Geometry check sheet. Reference: the model listing, model coordinates, mm. A direction names the side the tool comes from. Give positions to 0.01 mm unless a question says otherwise; leave off trailing zeros. Loops run counter-clockwise (first coordinate to the right, second up) from the corner with the lowest first, then second, coordinate; pieces in that order, holes last.
1. Cross-section at B-B, the plane y = -11. Record the cut outline in (x, z), plus the area to 3 significant figures.
2. Go/stop test with a flat-tipped pin: pin 1 Ø5 at (y, z) = (2, -0.5) entering from -X. Record where the tip stops, or that it passes through.
3. Cross-section at A-A, the plane x = -0.75. Record the cut outline in (y, z), plus the area to 3 significant figures.
4. Material ranges on L1, parallel to Z at x = 5.75, y = -11; L2, parallel to Z at x = -6.5, y = -8.8; L3, parallel to Y at x = -8.75, z = 3.75, recorded low to high.
5. Tool access check on faces 5 (the cylindrical face through (-5.633, 11.528, -3.905)), 6 (the cylindrical face through (3.79, -9.5, -5.93)), 7 (the flat face through (-5, -9.5, 3)), 8 (the flat face through (4, 13.5, 0)), 9 (the flat face through (0, 0, 0)). Record the directions out of +Z, -Z, +X, -X, +Y, -Y that give a thin tool (end or side, any length) a straight path to the whole face; none if there is none.
6. Cross-section at C-C, the plane z = 6. Record the cut outline in (x, y), plus the area to 3 significant figures.
7. Release check for a two-part mould opening along Y. For faces 1 (the flat face through (-8, 9.5, 3)), 2 (the flat face through (-3, 8.5, 0)), 3 (the flat face through (19, 0, 0)), 4 (the cylindrical face through (3.79, -9.5, 6.07)) record: +Y half, -Y half, draft (parallel to the pull), parting line (faces both ways), or undercut.
8. Cross-section at D-D, the plane x = 8. Record the cut outline in (y, z).
from build123d import *

# Parameters (mm, degrees)
F1_DEPTH = 8.5
F2_R     = 3
F3_DEPTH = 5
F2_R_2   = 4
F4_DEPTH = 4
F5_R     = 3
F6_DEPTH = 5
F5_R_2   = 4
F7_DEPTH = 4
F9_D     = 3


with BuildPart() as f1:
    # F0 (on Top) → F1 (new body, symmetric)
    with BuildSketch(Plane.XY):
        Polygon((19, 13.5), (-11, 13.5), (-11, 8.5), (0, 8.5), (0, -8.5), (-11, -8.5), (-11, -13.5), (19, -13.5), align=None)
    extrude(amount=F1_DEPTH, both=True)

    # F2 (on face) → F3 (cut, through all)
    with BuildSketch(Plane.XZ.offset(13.5)):
        with Locations((-6.5, 0)):
            Circle(F2_R)
    extrude(amount=-F3_DEPTH, mode=Mode.SUBTRACT)

    # F2 (on face) → F4 (cut)
    with BuildSketch(Plane.XZ.offset(13.5)):
        with Locations((-6.5, 0)):
            Circle(F2_R_2)
        with Locations((-6.5, 0)):
            Circle(F2_R, mode=Mode.SUBTRACT)
    extrude(amount=-F4_DEPTH, mode=Mode.SUBTRACT)

    # F5 (on face) → F6 (cut, through all)
    with BuildSketch(Plane(origin=(0, 13.5, 0), x_dir=(-1, 0, 0), z_dir=(0, 1, 0))):
        with Locations((6.5, 0)):
            Circle(F5_R)
    extrude(amount=-F6_DEPTH, mode=Mode.SUBTRACT)

    # F5 (on face) → F7 (cut)
    with BuildSketch(Plane(origin=(0, 13.5, 0), x_dir=(-1, 0, 0), z_dir=(0, 1, 0))):
        with Locations((6.5, 0)):
            Circle(F5_R_2)
        with Locations((6.5, 0)):
            Circle(F5_R, mode=Mode.SUBTRACT)
    extrude(amount=-F7_DEPTH, mode=Mode.SUBTRACT)

    # F9 (through all)
    with Locations(Plane.YZ.offset(19)):
        with Locations((-11, 6), (-11, -6), (11, -6), (11, 6)):
            Hole(F9_D / 2)


solid = f1.part
Result:
1. outline: (-11, -8.5) - (19, -8.5) - (19, -7.5) - (-11, -7.5) - close; (-11, -4.5) - (19, -4.5) - (19, 4.5) - (-11, 4.5) - close; (-11, 7.5) - (19, 7.5) - (19, 8.5) - (-11, 8.5) - close; hole circle Ø8 at (-6.5, 0)
1. area: 280 mm2
2. pin 1: stops at x = 0
3. outline: (-13.5, -8.5) - (-8.5, -8.5) - (-8.5, 8.5) - (-13.5, 8.5) - close; (8.5, -8.5) - (13.5, -8.5) - (13.5, 8.5) - (8.5, 8.5) - close; hole circle Ø3 at (-11, -6); hole circle Ø3 at (-11, 6); hole circle Ø3 at (11, -6); hole circle Ø3 at (11, 6)
3. area: 142 mm2
4. L1: z = -8.5 to -7.5, -4.5 to 4.5, 7.5 to 8.5
4. L2: z = -8.5 to -3, 3 to 8.5
4. L3: y = -13.5 to -8.5, 8.5 to 13.5
5. face 5: +Y
5. face 6: +X, -X
5. face 7: -Y
5. face 8: +Z, -Z, +X, -X, +Y
5. face 9: +Z, -Z, -X
6. outline: (-11, -13.5) - (19, -13.5) - (19, -12.5) - (-11, -12.5) - close; (-11, -9.5) - (19, -9.5) - (19, 9.5) - (-11, 9.5) - (-11, 8.5) - (0, 8.5) - (0, -8.5) - (-11, -8.5) - close; (-11, 12.5) - (19, 12.5) - (19, 13.5) - (-11, 13.5) - close
6. area: 443 mm2
7. face 1: +Y half
7. face 2: undercut
7. face 3: draft
7. face 4: undercut
8. outline: (-13.5, -8.5) - (13.5, -8.5) - (13.5, 8.5) - (-13.5, 8.5) - close; hole circle Ø3 at (-11, -6); hole circle Ø3 at (-11, 6); hole circle Ø3 at (11, -6); hole circle Ø3 at (11, 6)
